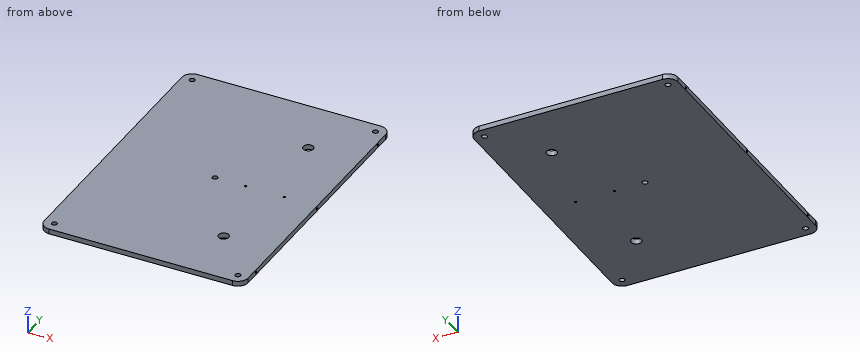
Autodesk Inventor part; units mm, degrees
ref_plane "YZ Plane" through (0, 0, 0) normal (1, 0, 0) x (0, 1, 0)
ref_plane "XZ Plane" through (0, 0, 0) normal (0, 1, 0) x (-1, 0, 0)
ref_plane "XY Plane" through (0, 0, 0) normal (0, 0, 1) x (1, 0, 0)
sketch "Sketch1" plane through (0, 0, 0) normal (0, 0, 1) x (1, 0, 0)
  line L0 (-127, 177.8) -> (127, 177.8)
  line L1 (127, 177.8) -> (127, -177.8)
  line L2 (127, -177.8) -> (-127, -177.8)
  line L3 (-127, -177.8) -> (-127, 177.8)
  point P0 (0, 0)
  dimension "d0" = 254
  dimension "d1" = 127
  dimension "d2" = 355.6
  dimension "d3" = 177.8
extrude "Extrusion1" add sketch "Sketch1" along normal blind 6.35
sketch "Sketch2" plane through (0, 0, 6.35) normal (0, 0, 1) x (1, 0, 0)
  line L0 (-114.3, 165.1) -> (114.3, 165.1) construction
  line L1 (114.3, 165.1) -> (114.3, -165.1) construction
  line L2 (114.3, -165.1) -> (-114.3, -165.1) construction
  line L3 (-114.3, -165.1) -> (-114.3, 165.1) construction
  line L4 (-127, 177.8) -> (127, 177.8) construction
  line L5 (127, -177.8) -> (-127, -177.8) construction
  line L6 (-127, -177.8) -> (-127, 177.8) construction
  line L7 (127, 177.8) -> (127, -177.8) construction
  point P0 (0, 0)
  point P1 (0, 0)
  dimension "d6" = 12.7
  dimension "d7" = 12.7
  dimension "d8" = 12.7
  dimension "d9" = 12.7
hole "Hole1" at (-114.3, 165.1, 6.35) at (114.3, 165.1, 6.35) at (114.3, -165.1, 6.35) at (-114.3, -165.1, 6.35) at (0, 0, 6.35) direction (0, 0, -1) diameter 6.7564 end through all
fillet "Fillet1" radius 12.7 4 edges at (127, -177.8, 3.175) (-127, -177.8, 3.175) (127, 177.8, 3.175) (-127, 177.8, 3.175)
sketch "Sketch9" plane through (127, -165.1, 0) normal (1, 0, 0) x (0, 0, -1)
  line L0 (-6.35, 330.2) -> (0, 330.2)
  line L1 (-6.35, 330.2) -> (-6.35, 0)
  line L2 (0, 0) -> (-6.35, 0)
  line L3 (0, 330.2) -> (0, 0)
  line L4 (-3.175, 330.2) -> (-3.175, 0) construction
  line L5 (0, 165.1) -> (-6.35, 165.1) construction
  point P0 (-3.175, 165.1)
  point P1 (-3.175, 311.15)
  point P2 (-3.175, 19.05)
  dimension "d68" = 146.05
hole "Hole6" at (127, 0, 3.175) at (127, 146.05, 3.175) at (127, -146.05, 3.175) direction (-1, 0, 0) diameter 2.6416 depth 15.24 tip angle 118
mirror "Mirror2" about plane through (0, 0, 0) normal (1, 0, 0) of "Hole6"
sketch "Sketch10" plane through (0, 0, 6.35) normal (0, 0, 1) x (1, 0, 0)
  line L0 (-177.8, 0) -> (177.8, 0) construction
  point P0 (0, 0)
  point P1 (86.36, 0)
  point P2 (38.1, 0)
  dimension "d76" = 48.26
  dimension "d85" = 38.1
hole "Hole7" at (86.36, 0, 6.35) at (38.1, 0, 6.35) direction (0, 0, -1) diameter 2.6416 end through all
sketch "Sketch11" plane through (0, 0, 6.35) normal (0, 0, 1) x (1, 0, 0)
  circle A0 centre (38.1, 0) radius 1.3208
  circle A1 centre (86.36, 0) radius 1.3208
  arc A2 (-114.3, 177.8) -> (-127, 165.1) centre (-114.3, 165.1) ccw
  line L0 (-127, -165.1) -> (-127, 165.1)
  arc A3 (-127, -165.1) -> (-114.3, -177.8) centre (-114.3, -165.1) ccw
  line L1 (114.3, -177.8) -> (-114.3, -177.8)
  arc A4 (114.3, -177.8) -> (127, -165.1) centre (114.3, -165.1) ccw
  line L2 (127, 165.1) -> (127, -165.1)
  arc A5 (127, 165.1) -> (114.3, 177.8) centre (114.3, 165.1) ccw
  line L3 (-114.3, 177.8) -> (114.3, 177.8)
  circle A6 centre (0, 0) radius 3.3782
  circle A7 centre (-114.3, -165.1) radius 3.3782
  circle A8 centre (114.3, -165.1) radius 3.3782
  circle A9 centre (114.3, 165.1) radius 3.3782
  circle A10 centre (-114.3, 165.1) radius 3.3782
  line L4 (63.5, 177.8) -> (63.5, -177.8) construction
  line L5 (-127, 0) -> (127, 0) construction
  point P0 (63.5, 101.6)
  point P1 (63.5, -101.6)
  dimension "d86" = 63.5
  dimension "d87" = 101.6
hole "Hole8" at (63.5, 101.6, 6.35) at (63.5, -101.6, 6.35) direction (0, 0, -1) diameter 12.7 end through all
properties part number "J001398" material "ALUMINUM, 6061-T651"
The listing builds one solid part. Answer for the finished solid, in the listing's coordinates (mm). Round coordinates to 2 decimals unless told otherwise and drop trailing zeros. Write each loop counter-clockwise with the first axis right and the second up, starting at its lowest first coordinate (ties: lowest second). Pieces come first, ordered by that corner, then holes. Notation, with made-up numbers: M 88.5,11.5 L 96.5,11.5 A26 cw 96.5,30.5 Z; hole C 56.5,32 d4. An arc over 180 degrees is marked long. Write each question's results on one line, items separated by ' | '. Start each with the question number.
Item 1: Flat-ended cylindrical pins translate along their axes: pin 1 Ø2 at (x, y) = (38.1, 0) entering from -Z; pin 2 Ø1.6 at (y, z) = (-146.05, 3.175) entering from -X; pin 3 Ø1.6 at (y, z) = (0, 3.175) entering from +X. Find the tip coordinate at first contact, or state that the pin passes through.
Item 2: A cutting plane is placed at A-A on x = 63.5. Write down the section's boundary in (y, z), and give its area (3 significant figures).
Item 3: Straight lines are drawn through the part: L1, parallel to Y at x = 114.3, z = 1.75; L2, parallel to Y at x = 63.5, z = 3.25; L3, parallel to Y at x = 0, z = 2.25. For each, find the intervals that lie inside material, in ascending order. Write a range as [from, to].
Check sheet entries:
1) pin 1: through | pin 2: x = -111.45 | pin 3: x = 111.45
2) outline: M -177.8,0 L -107.95,0 L -107.95,6.35 L -177.8,6.35 Z; M -95.25,0 L 95.25,0 L 95.25,6.35 L -95.25,6.35 Z; M 107.95,0 L 177.8,0 L 177.8,6.35 L 107.95,6.35 Z | area: 2,100 mm²
3) L1: [-177.8, -168.48], [-161.72, 161.72], [168.48, 177.8] | L2: [-177.8, -107.95], [-95.25, 95.25], [107.95, 177.8] | L3: [-177.8, -3.38], [3.38, 177.8]
